```python
from build123d import *

# Parameters (mm, degrees)
F1_DEPTH = 84
F3_DEPTH = 25
F4_R     = 7
F5_R     = 17.5
F6_DEPTH = 100


with BuildPart() as f1:
    # F0 (on Front) → F1 (new body)
    with BuildSketch(Plane.XZ):
        Polygon((-81.6743281484, 77.9422863406), (-36.6743281484, 0), (128.3256718516, 0), (128.3256718516, 23), (82.3256718516, 23), (44.7320598074, 23), (34.339754962, 41), (-10.660245038, 118.9422863406), (-27.9807531137, 108.9422863406), (17.0192468863, 31), (-19.3538200727, 10), (-64.3538200727, 87.9422863406), align=None)
    extrude(amount=F1_DEPTH)

    # F2 (on face) → F3 (cut)
    with BuildSketch(Plane.XY.offset(23)):
        with BuildLine():
            Line((128.3256718516, -27), (82.3256718516, -27))
            ThreePointArc((82.3256718516, -27), (67.3256718516, -42), (82.3256718516, -57))
            Line((82.3256718516, -57), (128.3256718516, -57))
            Line((128.3256718516, -57), (128.3256718516, -27))
        make_face()
    extrude(amount=-F3_DEPTH, mode=Mode.SUBTRACT)

    # F4
    f4_edges = [f1.edges().sort_by_distance(p)[0] for p in [
        (128.325672, 0, 11.5),
        (128.325672, -84, 11.5),
    ]]
    fillet(f4_edges, radius=F4_R)

    # F5 (on face) → F6 (cut)
    with BuildSketch(Plane(origin=(43.5083369991, 0, 25.1195500784), x_dir=(0, 1, 0), z_dir=(0.8660254038, 0, 0.5))):
        with Locations((-42, 66.3371640742)):
            Circle(F5_R)
        with BuildLine():
            ThreePointArc((-84, 66.3371640742), (-71.6984848098, 96.035648884), (-42, 108.3371640742))
            Line((-42, 108.3371640742), (-84, 108.3371640742))
            Line((-84, 108.3371640742), (-84, 66.3371640742))
        make_face()
        with BuildLine():
            ThreePointArc((-42, 108.3371640742), (-12.3015151902, 96.035648884), (0, 66.3371640742))
            Line((0, 66.3371640742), (0, 108.3371640742))
            Line((0, 108.3371640742), (-42, 108.3371640742))
        make_face()
    extrude(amount=-F6_DEPTH, mode=Mode.SUBTRACT)


solid = f1.part
```
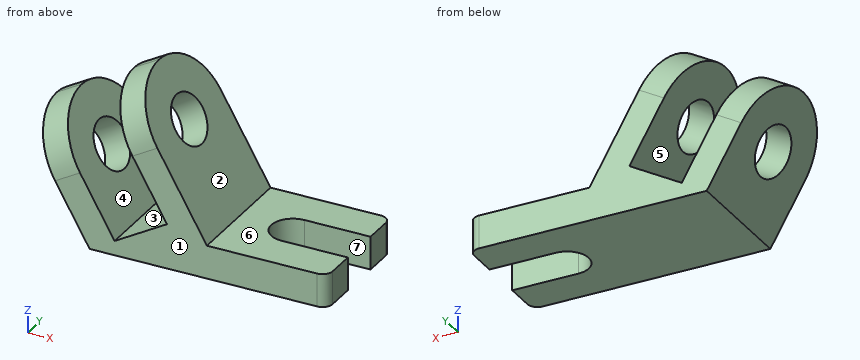
The model under review builds one solid part; all positions refer to its coordinate system, in mm. Face numbers are marked on the shaded views. A direction names the side the tool comes from. Round coordinates to 2 decimals unless told otherwise and drop trailing zeros. Order: outer loops, then holes, each group sorted by start corner. A loop starts at its lowest first (then second) coordinate and runs counter-clockwise, first axis right, second up.
(1) Take a section at C-C, the plane x = 73.5. State the section outline as (y, z) points.
Working result:
outline: (-84, 0) - (-54.13, 0) - (-54.13, 23) - (-84, 23) - close; (-29.87, 0) - (0, 0) - (0, 23) - (-29.87, 23) - close
(2) Mouldability with a two-part tool opening along X and no side actions: class the marked faces 1, 2, 3 and 4 as released by +X, released by -X, zero draft, split by the parting line, or undercut.
Working result:
face 1: zero draft
face 2: released by +X
face 3: undercut
face 4: undercut
(3) Take a section at A-A, the plane x = 108.5. State the section outline as (y, z) points.
Working result:
outline: (-84, 0) - (-57, 0) - (-57, 23) - (-84, 23) - close; (-27, 0) - (0, 0) - (0, 23) - (-27, 23) - close
(4) Wall thickness on L1, parallel to Z at x = 84.5, y = -18.5; L2, parallel to Z at x = 13, y = -41.5; L3, parallel to X at y = -66.5, z = 18.5: over which ranges is each line inside the solid? List them lowest first.
Working result:
L1: z = 0 to 23
L2: z = 0 to 28.68, 37.96 to 63.91
L3: x = -47.36 to -24.26, -4.63 to 128.33
(5) For P1, Ø12, axis at x = -43.5, y = -19.5, coming from the -Z side; P2, Ø12, axis at y = -72.5, z = 49, coming from the -X side; P3, Ø12, axis at y = -64.5, z = 21.5, coming from the -X side, all flat-tipped, find the tip position at first contact; note any pin that passes through.
Working result:
P1: stops at z = 1.43
P2: stops at x = -68.43
P3: stops at x = -52.55
(6) Tool access review of the marked faces 5, 6 and 7: name each direction out of +Z, -Z, +X, -X, +Y, -Y from which nothing blocks a thin tool from reaching the whole face with its end or side.
Working result:
face 5: +Y, -Y
face 6: +Z, +X, +Y, -Y
face 7: +Z, -Z, +X
(7) Take a section at B-B, the plane y = -47. State the section outline as (x, z) points (1 decimal), plus the area to 3 significant figures.
Working result:
outline: (-81.5, 77.7) - (-69.1, 56.1) - (-51.7, 66.1) - (-64.2, 87.7) - close; (-52.3, 27) - (-36.7, 0) - (68.2, 0) - (68.2, 23) - (44.7, 23) - (18.7, 68) - (1.4, 58) - (17, 31) - (-19.4, 10) - (-35, 37) - close; (-27.8, 108.7) - (-15.4, 87.1) - (2, 97.1) - (-10.5, 118.7) - close
area: 4,570 mm2
